```python
from build123d import *

# Parameters (mm, degrees)
SKETCH_1_W          = 50
SKETCH_1_H          = 19
SKETCH_1_R          = 1
EXTRUDE_1_DEPTH     = 2
SKETCH_2_R          = 0.75
SKETCH_2_R_2        = 0.5
CUT_EXTRUDE_1_DEPTH = 2
CHAMFER_1_SIZE      = 0.25


with BuildPart() as part:
    # Эскиз1 → Бобышка-Вытянуть1 (new body)
    with BuildSketch(Plane.XY):
        Rectangle(SKETCH_1_W, SKETCH_1_H)
        with Locations((-22.5, 7)):
            Circle(SKETCH_1_R, mode=Mode.SUBTRACT)
        with Locations((22.5, 7)):
            Circle(SKETCH_1_R, mode=Mode.SUBTRACT)
        with Locations((22.5, -7)):
            Circle(SKETCH_1_R, mode=Mode.SUBTRACT)
        with Locations((-22.5, -7)):
            Circle(SKETCH_1_R, mode=Mode.SUBTRACT)
    extrude(amount=EXTRUDE_1_DEPTH)

    # Эскиз2 → Вырез-Вытянуть1 (cut)
    with BuildSketch(Plane.XY.offset(2)):
        with Locations((-5.7, 6)):
            Circle(SKETCH_2_R)
        with Locations((-5.7, -6)):
            Circle(SKETCH_2_R)
        with Locations((6.5, 6)):
            Circle(SKETCH_2_R)
        with Locations((6.5, -6)):
            Circle(SKETCH_2_R)
        with Locations((8.5, 0)):
            Circle(SKETCH_2_R)
        with Locations((16, 2.5)):
            Circle(SKETCH_2_R)
        with Locations((16, -2.5)):
            Circle(SKETCH_2_R)
        with Locations((14.75, 7)):
            Circle(SKETCH_2_R_2)
        with Locations((-20, 0.7)):
            Circle(SKETCH_2_R)
        with Locations((-15, 0.7)):
            Circle(SKETCH_2_R)
        with Locations((17.25, 7)):
            Circle(SKETCH_2_R_2)
    extrude(amount=-CUT_EXTRUDE_1_DEPTH, mode=Mode.SUBTRACT)

    # Фаска1
    chamfer_1_edges = [part.edges().sort_by_distance(p)[0] for p in [
        (-25, 0, 2),
        (0, -9.5, 2),
        (25, 0, 2),
        (0, -9.5, 0),
        (-25, 0, 0),
        (0, 9.5, 0),
        (25, 0, 0),
        (0, 9.5, 2),
        (25, -9.5, 1),
        (-25, -9.5, 1),
        (-25, 9.5, 1),
        (25, 9.5, 1),
    ]]
    chamfer(chamfer_1_edges, length=CHAMFER_1_SIZE)


solid = part.part
```
Could you check a few things on this model? Use its own coordinates, in mm. Give positions to 0.01 mm unless a question says otherwise; leave off trailing zeros. Loops run counter-clockwise (first coordinate to the right, second up) from the corner with the lowest first, then second, coordinate; pieces in that order, holes last. Notation, with made-up numbers: (77.5, 62) - (121.5, 62) arc R11 cw to (121.5, 80) - close; hole circle Ø6 at (-19.5, 34). An arc over 180 degrees is marked (long way). Answer in a Markdown table with one row per item. Add a question column.
Q1. For pin 1 (1.2 mm diameter, centred on x = -5.7, y = -6, fed in from +Z), with a flat end and sliding along its axis, tell me the tip position at first contact or that it passes through.
Q2. We'd pull the mould along Y, two halves only. Please class faces 1 (the face through (14.981, 6.556, 1.014)), 2 (the face through (0, 9.5, 1)), 3 (the face through (25, 0, 1)): +Y half, -Y half, draft (parallel to the pull), parting line (faces both ways), or undercut.
Q3. Please list where these lines run through material, in increasing order: L1, parallel to Y at x = 14.75, z = 1; L2, parallel to X at y = 5.5, z = 0.55; L3, parallel to X at y = 0.5, z = 0.1. Write a range as from..to.
Q4. If we section it at C-C (x = 22.5): List the corners of the cut face in (y, z) for me.
Q5. If we section it at A-A (x = 6.5): List the corners of the cut face in (y, z) for me, plus the area to 3 significant figures.
Q6. If we section it at B-B (x = -15): List the corners of the cut face in (y, z) for me, plus the area to 3 significant figures.
The answers:
| question | item | result |
|---|---|---|
| 1 | pin 1 | passes through |
| 2 | face 1 | undercut |
| 2 | face 2 | +Y half |
| 2 | face 3 | draft |
| 3 | L1 | y = -9.5..6.5, 7.5..9.5 |
| 3 | L2 | x = -25..-6.26, -5.14..5.94, 7.06..25 |
| 3 | L3 | x = -24.85..-20.72, -19.28..-15.72, -14.28..7.94, 9.06..24.85 |
| 4 | outline | (-9.5, 0.25) - (-9.25, 0) - (-8, 0) - (-8, 2) - (-9.25, 2) - (-9.5, 1.75) - close; (-6, 0) - (6, 0) - (6, 2) - (-6, 2) - close; (8, 0) - (9.25, 0) - (9.5, 0.25) - (9.5, 1.75) - (9.25, 2) - (8, 2) - close |
| 5 | outline | (-9.5, 0.25) - (-9.25, 0) - (-6.75, 0) - (-6.75, 2) - (-9.25, 2) - (-9.5, 1.75) - close; (-5.25, 0) - (5.25, 0) - (5.25, 2) - (-5.25, 2) - close; (6.75, 0) - (9.25, 0) - (9.5, 0.25) - (9.5, 1.75) - (9.25, 2) - (6.75, 2) - close |
| 5 | area | 31.9 mm^2 |
| 6 | outline | (-9.5, 0.25) - (-9.25, 0) - (-0.05, 0) - (-0.05, 2) - (-9.25, 2) - (-9.5, 1.75) - close; (1.45, 0) - (9.25, 0) - (9.5, 0.25) - (9.5, 1.75) - (9.25, 2) - (1.45, 2) - close |
| 6 | area | 34.9 mm^2 |
